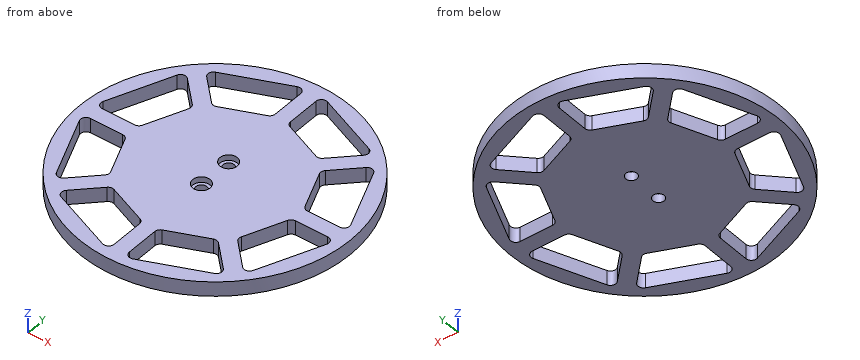
from build123d import *

# Parameters (mm, degrees)
SKETCH1_R           = 74.25
SKETCH1_R_2         = 3.05
BOSS_EXTRUDE1_DEPTH = 8
SKETCH2_R           = 4.75
CUT_EXTRUDE1_DEPTH  = 3.1


with BuildPart() as part:
    # Sketch1 → Boss-Extrude1 (new body)
    with BuildSketch(Plane.XY):
        Circle(SKETCH1_R)
        with Locations((0, 9.5)):
            Circle(SKETCH1_R_2, mode=Mode.SUBTRACT)
        with Locations((0, -9.5)):
            Circle(SKETCH1_R_2, mode=Mode.SUBTRACT)
        with BuildLine():
            Line((67.925889957, 8.348050297), (53.933820381, 42.127894432))
            ThreePointArc((53.933820381, 42.127894432), (51.74745275, 43.922199976), (49.04086144, 43.101164478))
            Line((49.04086144, 43.101164478), (36.488844859, 30.549147897))
            ThreePointArc((36.488844859, 30.549147897), (35.667809361, 29.013098519), (35.838526605, 27.279777256))
            Line((35.838526605, 27.279777256), (44.631380677, 6.051949703))
            ThreePointArc((44.631380677, 6.051949703), (45.736308575, 4.705591163), (47.403019275, 4.2))
            Line((47.403019275, 4.2), (65.154251359, 4.2))
            ThreePointArc((65.154251359, 4.2), (67.648660196, 5.533289301), (67.925889957, 8.348050297))
        make_face(mode=Mode.SUBTRACT)
        with BuildLine():
            Line((42.127894432, 53.933820381), (8.348050297, 67.925889957))
            ThreePointArc((8.348050297, 67.925889957), (5.533289301, 67.648660196), (4.2, 65.154251359))
            Line((4.2, 65.154251359), (4.2, 47.403019275))
            ThreePointArc((4.2, 47.403019275), (4.705591163, 45.736308575), (6.051949703, 44.631380677))
            Line((6.051949703, 44.631380677), (27.279777256, 35.838526605))
            ThreePointArc((27.279777256, 35.838526605), (29.013098519, 35.667809361), (30.549147897, 36.488844859))
            Line((30.549147897, 36.488844859), (43.101164478, 49.04086144))
            ThreePointArc((43.101164478, 49.04086144), (43.922199976, 51.74745275), (42.127894432, 53.933820381))
        make_face(mode=Mode.SUBTRACT)
        with BuildLine():
            Line((-8.348050297, 67.925889957), (-42.127894432, 53.933820381))
            ThreePointArc((-42.127894432, 53.933820381), (-43.922199976, 51.74745275), (-43.101164478, 49.04086144))
            Line((-43.101164478, 49.04086144), (-30.549147897, 36.488844859))
            ThreePointArc((-30.549147897, 36.488844859), (-29.013098519, 35.667809361), (-27.279777256, 35.838526605))
            Line((-27.279777256, 35.838526605), (-6.051949703, 44.631380677))
            ThreePointArc((-6.051949703, 44.631380677), (-4.705591163, 45.736308575), (-4.2, 47.403019275))
            Line((-4.2, 47.403019275), (-4.2, 65.154251359))
            ThreePointArc((-4.2, 65.154251359), (-5.533289301, 67.648660196), (-8.348050297, 67.925889957))
        make_face(mode=Mode.SUBTRACT)
        with BuildLine():
            Line((-53.933820381, 42.127894432), (-67.925889957, 8.348050297))
            ThreePointArc((-67.925889957, 8.348050297), (-67.648660196, 5.533289301), (-65.154251359, 4.2))
            Line((-65.154251359, 4.2), (-47.403019275, 4.2))
            ThreePointArc((-47.403019275, 4.2), (-45.736308575, 4.705591163), (-44.631380677, 6.051949703))
            Line((-44.631380677, 6.051949703), (-35.838526605, 27.279777256))
            ThreePointArc((-35.838526605, 27.279777256), (-35.667809361, 29.013098519), (-36.488844859, 30.549147897))
            Line((-36.488844859, 30.549147897), (-49.04086144, 43.101164478))
            ThreePointArc((-49.04086144, 43.101164478), (-51.74745275, 43.922199976), (-53.933820381, 42.127894432))
        make_face(mode=Mode.SUBTRACT)
        with BuildLine():
            Line((-67.925889957, -8.348050297), (-53.933820381, -42.127894432))
            ThreePointArc((-53.933820381, -42.127894432), (-51.74745275, -43.922199976), (-49.04086144, -43.101164478))
            Line((-49.04086144, -43.101164478), (-36.488844859, -30.549147897))
            ThreePointArc((-36.488844859, -30.549147897), (-35.667809361, -29.013098519), (-35.838526605, -27.279777256))
            Line((-35.838526605, -27.279777256), (-44.631380677, -6.051949703))
            ThreePointArc((-44.631380677, -6.051949703), (-45.736308575, -4.705591163), (-47.403019275, -4.2))
            Line((-47.403019275, -4.2), (-65.154251359, -4.2))
            ThreePointArc((-65.154251359, -4.2), (-67.648660196, -5.533289301), (-67.925889957, -8.348050297))
        make_face(mode=Mode.SUBTRACT)
        with BuildLine():
            Line((-42.127894432, -53.933820381), (-8.348050297, -67.925889957))
            ThreePointArc((-8.348050297, -67.925889957), (-5.533289301, -67.648660196), (-4.2, -65.154251359))
            Line((-4.2, -65.154251359), (-4.2, -47.403019275))
            ThreePointArc((-4.2, -47.403019275), (-4.705591163, -45.736308575), (-6.051949703, -44.631380677))
            Line((-6.051949703, -44.631380677), (-27.279777256, -35.838526605))
            ThreePointArc((-27.279777256, -35.838526605), (-29.013098519, -35.667809361), (-30.549147897, -36.488844859))
            Line((-30.549147897, -36.488844859), (-43.101164478, -49.04086144))
            ThreePointArc((-43.101164478, -49.04086144), (-43.922199976, -51.74745275), (-42.127894432, -53.933820381))
        make_face(mode=Mode.SUBTRACT)
        with BuildLine():
            Line((8.348050297, -67.925889957), (42.127894432, -53.933820381))
            ThreePointArc((42.127894432, -53.933820381), (43.922199976, -51.74745275), (43.101164478, -49.04086144))
            Line((43.101164478, -49.04086144), (30.549147897, -36.488844859))
            ThreePointArc((30.549147897, -36.488844859), (29.013098519, -35.667809361), (27.279777256, -35.838526605))
            Line((27.279777256, -35.838526605), (6.051949703, -44.631380677))
            ThreePointArc((6.051949703, -44.631380677), (4.705591163, -45.736308575), (4.2, -47.403019275))
            Line((4.2, -47.403019275), (4.2, -65.154251359))
            ThreePointArc((4.2, -65.154251359), (5.533289301, -67.648660196), (8.348050297, -67.925889957))
        make_face(mode=Mode.SUBTRACT)
        with BuildLine():
            Line((53.933820381, -42.127894432), (67.925889957, -8.348050297))
            ThreePointArc((67.925889957, -8.348050297), (67.648660196, -5.533289301), (65.154251359, -4.2))
            Line((65.154251359, -4.2), (47.403019275, -4.2))
            ThreePointArc((47.403019275, -4.2), (45.736308575, -4.705591163), (44.631380677, -6.051949703))
            Line((44.631380677, -6.051949703), (35.838526605, -27.279777256))
            ThreePointArc((35.838526605, -27.279777256), (35.667809361, -29.013098519), (36.488844859, -30.549147897))
            Line((36.488844859, -30.549147897), (49.04086144, -43.101164478))
            ThreePointArc((49.04086144, -43.101164478), (51.74745275, -43.922199976), (53.933820381, -42.127894432))
        make_face(mode=Mode.SUBTRACT)
    extrude(amount=BOSS_EXTRUDE1_DEPTH)

    # Sketch2 → Cut-Extrude1 (cut)
    with BuildSketch(Plane.XY.offset(8)):
        with Locations((0, -9.5)):
            Circle(SKETCH2_R)
        with Locations((0, 9.5)):
            Circle(SKETCH2_R)
    extrude(amount=-CUT_EXTRUDE1_DEPTH, mode=Mode.SUBTRACT)


solid = part.part
Here's how the part is built. I have some questions about the finished solid (model axes, mm). Give positions to 0.01 mm unless a question says otherwise; leave off trailing zeros. Write each loop counter-clockwise with the first axis right and the second up, starting at its lowest first coordinate (ties: lowest second). Pieces come first, ordered by that corner, then holes. Notation, with made-up numbers: (-33, 31) -> (-4, 31) arc R9 cw to (-4, 37) -> close; hole circle Ø10 at (68.25, 9). An arc over 180 degrees is marked (long way). Use one line per item in the form item = value. Start each with the question number.
1. If I drill on L1, parallel to Y at x = 0, z = 7; L2, parallel to Y at x = 0, z = 2.25; L3, parallel to X at y = -9.5, z = 1.45, over which ranges is the centre line in solid material (lowest first)?
2. Imagine slicing it at B-B on z = 6.25. State how many separate pieces and enclosed holes the cut face has, plus the area to 3 significant figures.
3. Imagine slicing it at D-D on x = -33.5. List the corners of the cut face in (y, z) for me, plus the area to 3 significant figures.
4. Will these pins go through, and if not, where does the flat tip stop? pin 1 Ø1 at (x, y) = (24, 4) entering from -Z; pin 2 Ø2.5 at (x, z) = (53.5, 3) entering from -Y; pin 3 Ø4 at (x, z) = (-15, 5.5) entering from +Y; pin 4 Ø5 at (x, y) = (-1, -9) entering from +Z.
5. Imagine slicing it at C-C on y = 38.5. List the corners of the cut face in (x, z) for me.
6. Imagine slicing it at A-A on x = 0. List the corners of the cut face in (y, z) for me, plus the area to 3 significant figures.
Entries:
q1.L1 = -74.25 to -14.25, -4.75 to 4.75, 14.25 to 74.25
q1.L2 = -74.25 to -12.55, -6.45 to 6.45, 12.55 to 74.25
q1.L3 = -73.64 to -67.45, -43.2 to -3.05, 3.05 to 43.2, 67.45 to 73.64
q2.separate_pieces = 1
q2.enclosed_holes = 10
q2.area = 10,800 mm²
q3.outline = (-66.26, 0) -> (-57.51, 0) -> (-57.51, 8) -> (-66.26, 8) -> close; (-39.44, 0) -> (39.44, 0) -> (39.44, 8) -> (-39.44, 8) -> close; (57.51, 0) -> (66.26, 0) -> (66.26, 8) -> (57.51, 8) -> close
q3.area = 771 mm²
q4.pin_1 = 0
q4.pin_2 = -52.75
q4.pin_3 = 73.1
q4.pin_4 = 4.9
q5.outline = (-63.49, 0) -> (-55.44, 0) -> (-55.44, 8) -> (-63.49, 8) -> close; (-44.44, 0) -> (-32.56, 0) -> (-32.56, 8) -> (-44.44, 8) -> close; (-20.85, 0) -> (20.85, 0) -> (20.85, 8) -> (-20.85, 8) -> close; (32.56, 0) -> (44.44, 0) -> (44.44, 8) -> (32.56, 8) -> close; (55.44, 0) -> (63.49, 0) -> (63.49, 8) -> (55.44, 8) -> close
q6.outline = (-74.25, 0) -> (-12.55, 0) -> (-12.55, 4.9) -> (-14.25, 4.9) -> (-14.25, 8) -> (-74.25, 8) -> close; (-6.45, 0) -> (6.45, 0) -> (6.45, 4.9) -> (4.75, 4.9) -> (4.75, 8) -> (-4.75, 8) -> (-4.75, 4.9) -> (-6.45, 4.9) -> close; (12.55, 0) -> (74.25, 0) -> (74.25, 8) -> (14.25, 8) -> (14.25, 4.9) -> (12.55, 4.9) -> close
q6.area = 1,070 mm²
